The listing builds one solid part. Answer for the finished solid, in the listing's coordinates (mm). Give positions to 0.01 mm unless a question says otherwise; leave off trailing zeros. Write each loop counter-clockwise with the first axis right and the second up, starting at its lowest first coordinate (ties: lowest second). Pieces come first, ordered by that corner, then holes.
```python
from build123d import *

# Parameters (mm, degrees)
SKETCH_1_W          = 15
SKETCH_1_H          = 110
EXTRUDE_1_DEPTH     = 3
FILLET_1_R          = 1
SKETCH_2_R          = 1.25
CUT_EXTRUDE_1_DEPTH = 3
SKETCH_3_R          = 1.5
CUT_EXTRUDE_2_DEPTH = 10


with BuildPart() as part:
    # 草图1 → 凸台-拉伸1 (new body)
    with BuildSketch(Plane(origin=(0, 0, 0), x_dir=(1, 0, 0), z_dir=(0, 1, 0))):
        with Locations((7.5, 55)):
            Rectangle(SKETCH_1_W, SKETCH_1_H)
    extrude(amount=EXTRUDE_1_DEPTH)

    # 圆角1
    fillet_1_edges = [part.edges().sort_by_distance(p)[0] for p in [
        (0, 1.5, -110),
        (15, 1.5, -110),
        (15, 1.5, 0),
        (0, 1.5, 0),
    ]]
    fillet(fillet_1_edges, radius=FILLET_1_R)

    # 草图2 → 切除-拉伸1 (cut)
    with BuildSketch(Plane(origin=(0, 3, 0), x_dir=(1, 0, 0), z_dir=(0, 1, 0))):
        with Locations((7.5, 13)):
            Circle(SKETCH_2_R)
        with Locations((7.5, 57.5)):
            Circle(SKETCH_2_R)
    extrude(amount=-CUT_EXTRUDE_1_DEPTH, mode=Mode.SUBTRACT)

    # 草图3 → 切除-拉伸2 (cut)
    with BuildSketch(Plane(origin=(0, 3, 0), x_dir=(1, 0, 0), z_dir=(0, 1, 0))):
        with Locations((7.5, 40)):
            Circle(SKETCH_3_R)
        with Locations((7.5, 31)):
            Circle(SKETCH_3_R)
    extrude(amount=-CUT_EXTRUDE_2_DEPTH, mode=Mode.SUBTRACT)


solid = part.part
```
Item 1: A cutting plane is placed at A-A, the plane z = -31. Give the vertices of the cut face in (x, y).
Conclusion:
outline: (0, 0) - (6, 0) - (6, 3) - (0, 3) - close; (9, 0) - (15, 0) - (15, 3) - (9, 3) - close
Item 2: Consider probe 1 along Z at (x, y) = (7.5, 2.4); probe 2 along X at (y, z) = (0.95, -13); probe 3 along X at (y, z) = (2.2, -31). Determine where each line is inside the solid, lowest interval first.
Conclusion:
probe 1: z = -110 to -58.75, -56.25 to -41.5, -38.5 to -32.5, -29.5 to -14.25, -11.75 to 0
probe 2: x = 0 to 6.25, 8.75 to 15
probe 3: x = 0 to 6, 9 to 15
Item 3: A cutting plane is placed at B-B, the plane x = 7.5. Give the vertices of the cut face in (y, z), plus the area to 3 significant figures.
Conclusion:
outline: (0, -110) - (3, -110) - (3, -58.75) - (0, -58.75) - close; (0, -56.25) - (3, -56.25) - (3, -41.5) - (0, -41.5) - close; (0, -38.5) - (3, -38.5) - (3, -32.5) - (0, -32.5) - close; (0, -29.5) - (3, -29.5) - (3, -14.25) - (0, -14.25) - close; (0, -11.75) - (3, -11.75) - (3, 0) - (0, 0) - close
area: 297 mm2
Item 4: A cutting plane is placed at C-C, the plane y = 2.4. Give the vertices of the cut face in (x, z).
Conclusion:
outline: (0, -109) arc R1 ccw to (1, -110) - (14, -110) arc R1 ccw to (15, -109) - (15, -1) arc R1 ccw to (14, 0) - (1, 0) arc R1 ccw to (0, -1) - close; hole circle Ø3 at (7.5, -40); hole circle Ø3 at (7.5, -31); hole circle Ø2.5 at (7.5, -57.5); hole circle Ø2.5 at (7.5, -13)
Item 5: A cutting plane is placed at D-D, the plane z = -57.5. Give the vertices of the cut face in (x, y), plus the area to 3 significant figures.
Conclusion:
outline: (0, 0) - (6.25, 0) - (6.25, 3) - (0, 3) - close; (8.75, 0) - (15, 0) - (15, 3) - (8.75, 3) - close
area: 37.5 mm2
Item 6: Determine the mould class of faces 1 (the face through (6.579, 1.521, -13.845)), 2 (the face through (7, 0, -56)), 3 (the face through (0, 1, -54)) for opening direction X: pulls with the +X half, pulls with the -X half, needs draft (parallel to the pull), parting line crosses it, or undercut.
Conclusion:
face 1: undercut
face 2: needs draft
face 3: pulls with the -X half
